Part print with two shaded views. Sizes in mm from the minimum x, y, z corner. Round coordinates to 2 decimals unless told otherwise and drop trailing zeros. Loops run counter-clockwise (first coordinate to the right, second up) from the corner with the lowest first, then second, coordinate; pieces in that order, holes last.
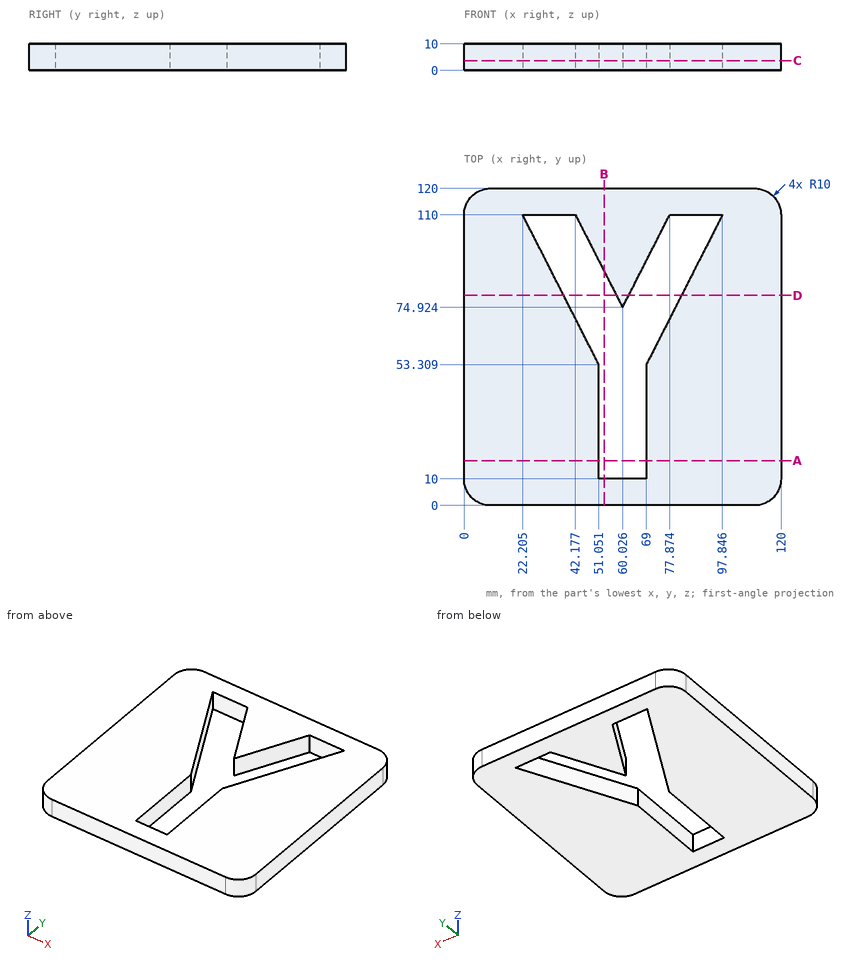
Item 1: Cut at D-D (y = 79.5). List the corners of the cut face in (x, z) (1 decimal).
Verdict:
outline: (0, 0) - (37.7, 0) - (37.7, 10) - (0, 10) - close; (57.7, 0) - (62.4, 0) - (62.4, 10) - (57.7, 10) - close; (82.3, 0) - (120, 0) - (120, 10) - (82.3, 10) - close
Item 2: Cut at B-B (x = 53). List the corners of the cut face in (y, z).
Verdict:
outline: (0, 0) - (10, 0) - (10, 10) - (0, 10) - close; (88.73, 0) - (120, 0) - (120, 10) - (88.73, 10) - close
Item 3: Wall check: L1, parallel to X at y = 11, z = 3.75; L2, parallel to X at y = 94, z = 4.5 (1 decimal); L3, parallel to X at y = 97, z = 7.75. Give the ranges that are in metal, low to high.
Verdict:
L1: x = 0 to 51.05, 69 to 120
L2: x = 0 to 30.3, 50.3 to 69.7, 89.7 to 120
L3: x = 0 to 28.82, 48.79 to 71.26, 91.23 to 120
Item 4: Cut at C-C (z = 3.75). List the corners of the cut face in (x, y) (1 decimal).
Verdict:
outline: (0, 10) arc R10 ccw to (10, 0) - (110, 0) arc R10 ccw to (120, 10) - (120, 110) arc R10 ccw to (110, 120) - (10, 120) arc R10 ccw to (0, 110) - close; hole (22.2, 110) - (51.1, 53.3) - (51.1, 10) - (69, 10) - (69, 53.3) - (97.8, 110) - (77.9, 110) - (60, 74.9) - (42.2, 110) - close
Item 5: Flat gauge pins, fed straight in: P1, Ø6, axis at y = 47.5, z = 2, coming from the -X side; P2, Ø10, axis at x = 59, y = 65, coming from the +Z side. Where does each tip first touch, or does it go through?
Verdict:
P1: stops at x = 0
P2: passes through
Item 6: Cut at A-A (y = 17). List the corners of the cut face in (x, z).
Verdict:
outline: (0, 0) - (51.05, 0) - (51.05, 10) - (0, 10) - close; (69, 0) - (120, 0) - (120, 10) - (69, 10) - close
